Part print with two shaded views. Sizes in mm from the minimum x, y, z corner. A direction names the side the tool comes from. Round coordinates to 2 decimals unless told otherwise and drop trailing zeros. Write each loop counter-clockwise with the first axis right and the second up, starting at its lowest first coordinate (ties: lowest second). Pieces come first, ordered by that corner, then holes. Notation, with made-up numbers: (51, 10) -> (86, 10) arc R20 ccw to (86, 25) -> close; hole circle Ø2 at (-39.75, -7). An arc over 180 degrees is marked (long way). Answer in a Markdown table with one row per item. Add a question column.
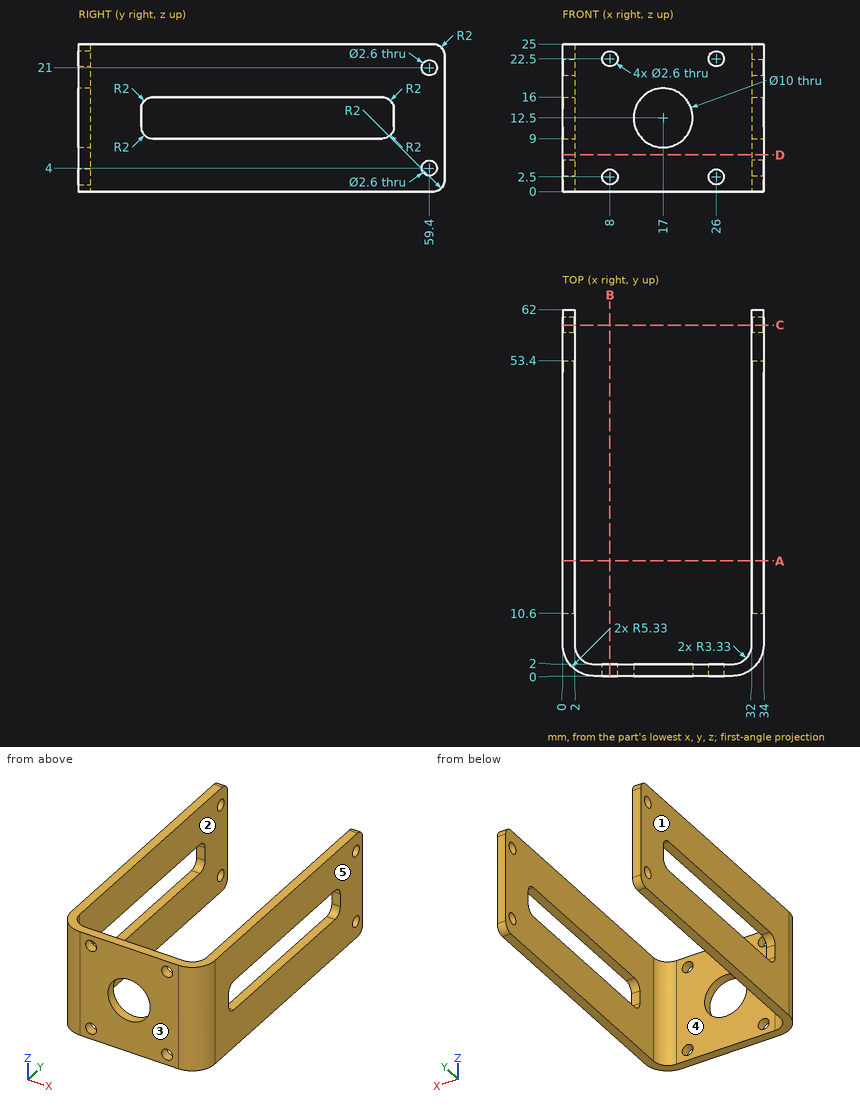
Item 1: Tool access for the marked faces 1 and 2: list every direction of +Z, -Z, +X, -X, +Y, -Y with a clear straight run to the whole face (end or side of a thin tool).
Item 2: Saw through at C-C on y = 59.4. Give the cut face in (x, z).
Item 3: Pin check, flat tips, straight feed: pin 1 (1.6 mm diameter, centred on x = 32.5, y = 37, fed in from -Z); pin 2 (3.5 mm diameter, centred on x = 8, z = 22.5, fed in from +Y); pin 3 (1 mm diameter, centred on x = 33, z = 12, fed in from -Y); pin 4 (1 mm diameter, centred on x = 0.5, z = 12.5, fed in from -Y). Stop position of each tip, or through.
Item 4: Two-plate mould, pull along X, no slides. Class the marked faces 3, 4 and 5: +X half, -X half, draft (parallel to the pull), parting line (faces both ways), or undercut.
Item 5: Saw through at B-B on x = 8. Give the cut face in (y, z).
Item 6: Saw through at A-A on y = 19.5. Give the cut face in (x, z).
Item 7: Drill centre lines: probe 1 along X at (y, z) = (30, 4.5); probe 2 along Z at (x, y) = (33.1, 59.4); probe 3 along X at (y, z) = (0.6, 2.5). Where is each one in solid material? Low to high.
Item 8: Saw through at D-D on z = 6.25. Give the cut face in (x, y).
Recorded:
| question | item | result |
|---|---|---|
| 1 | face 1 | +Z, -Z, -X, +Y, -Y |
| 1 | face 2 | +Z, -Z, +Y |
| 2 | outline | (0, 0) -> (2, 0) -> (2, 2.7) -> (0, 2.7) -> close; (0, 5.3) -> (2, 5.3) -> (2, 19.7) -> (0, 19.7) -> close; (0, 22.3) -> (2, 22.3) -> (2, 25) -> (0, 25) -> close; (32, 0) -> (34, 0) -> (34, 2.7) -> (32, 2.7) -> close; (32, 5.3) -> (34, 5.3) -> (34, 19.7) -> (32, 19.7) -> close; (32, 22.3) -> (34, 22.3) -> (34, 25) -> (32, 25) -> close |
| 3 | pin 1 | z = 0 |
| 3 | pin 2 | y = 2 |
| 3 | pin 3 | y = 1.62 |
| 3 | pin 4 | y = 2.22 |
| 4 | face 3 | draft |
| 4 | face 4 | undercut |
| 4 | face 5 | +X half |
| 5 | outline | (0, 0) -> (2, 0) -> (2, 1.2) -> (0, 1.2) -> close; (0, 3.8) -> (2, 3.8) -> (2, 21.2) -> (0, 21.2) -> close; (0, 23.8) -> (2, 23.8) -> (2, 25) -> (0, 25) -> close |
| 6 | outline | (0, 0) -> (2, 0) -> (2, 9) -> (0, 9) -> close; (0, 16) -> (2, 16) -> (2, 25) -> (0, 25) -> close; (32, 0) -> (34, 0) -> (34, 9) -> (32, 9) -> close; (32, 16) -> (34, 16) -> (34, 25) -> (32, 25) -> close |
| 7 | probe 1 | 0 to 2, 32 to 34 |
| 7 | probe 2 | 0 to 2.7, 5.3 to 19.7, 22.3 to 25 |
| 7 | probe 3 | 2.87 to 6.7, 9.3 to 24.7, 27.3 to 31.13 |
| 8 | outline | (0, 5.33) arc R5.33 ccw to (5.33, 0) -> (28.67, 0) arc R5.33 ccw to (34, 5.33) -> (34, 62) -> (32, 62) -> (32, 5.33) arc R3.33 cw to (28.67, 2) -> (5.33, 2) arc R3.33 cw to (2, 5.33) -> (2, 62) -> (0, 62) -> close |
